```python
from build123d import *

# Parameters (mm, degrees)
SKETCH1_R           = 133.35
BOSS_EXTRUDE1_DEPTH = 19.05
SKETCH2_R           = 3.6703
SKETCH2_R_2         = 2.5781
SKETCH2_R_3         = 1.7859375
CUT_EXTRUDE1_DEPTH  = 20.05
BOSS_EXTRUDE2_DEPTH = 19.05
FILLET1_R           = 25.4
SKETCH4_R           = 3.175
CUT_EXTRUDE2_DEPTH  = 20.05
SKETCH5_R           = 7.9375
CUT_EXTRUDE3_DEPTH  = 15.875
CUT_EXTRUDE4_DEPTH  = 20.05
CUT_EXTRUDE5_DEPTH  = 12.7
FILLET2_R           = 3.175
CUT_EXTRUDE6_DEPTH  = 3.175


with BuildPart() as part:
    # Sketch1 → Boss-Extrude1 (new body)
    with BuildSketch(Plane(origin=(0, 0, 0), x_dir=(1, 0, 0), z_dir=(0, 1, 0))):
        Circle(SKETCH1_R)
    extrude(amount=BOSS_EXTRUDE1_DEPTH)

    # Sketch2 → Cut-Extrude1 (cut, through all)
    with BuildSketch(Plane(origin=(0, 19.05, 0), x_dir=(1, 0, 0), z_dir=(0, 1, 0))):
        with Locations((-120.2563, 0)):
            Circle(SKETCH2_R)
        with Locations((-111.10233558, 46.02009338)):
            Circle(SKETCH2_R_2)
        with Locations((120.2563, 0)):
            Circle(SKETCH2_R)
        with Locations((0, -120.2563)):
            Circle(SKETCH2_R)
        with Locations((0, 120.2563)):
            Circle(SKETCH2_R)
        with Locations((111.10233558, -46.02009338)):
            Circle(SKETCH2_R_2)
        with Locations((-46.02009338, -111.10233558)):
            Circle(SKETCH2_R_2)
        with Locations((46.02009338, 111.10233558)):
            Circle(SKETCH2_R_2)
        with Locations((-85.03404521, -85.03404521)):
            Circle(SKETCH2_R_3)
        with Locations((85.03404521, 85.03404521)):
            Circle(SKETCH2_R_3)
        with Locations((-85.03404521, 85.03404521)):
            Circle(SKETCH2_R_3)
        with Locations((85.03404521, -85.03404521)):
            Circle(SKETCH2_R_3)
    extrude(amount=-CUT_EXTRUDE1_DEPTH, mode=Mode.SUBTRACT)

    # Sketch3 → Boss-Extrude2 (add)
    with BuildSketch(Plane(origin=(0, 19.05, 0), x_dir=(1, 0, 0), z_dir=(0, 1, 0))):
        with BuildLine():
            Line((-106.3625, 80.431592635), (-106.3625, 188.9125))
            ThreePointArc((-106.3625, 188.9125), (-102.642756121, 197.892756121), (-93.6625, 201.6125))
            Line((-93.6625, 201.6125), (93.6625, 201.6125))
            ThreePointArc((93.6625, 201.6125), (102.642756121, 197.892756121), (106.3625, 188.9125))
            Line((106.3625, 188.9125), (106.3625, 80.431592635))
            ThreePointArc((106.3625, 80.431592635), (0, 133.35), (-106.3625, 80.431592635))
        make_face()
    extrude(amount=-BOSS_EXTRUDE2_DEPTH)

    # Fillet1
    fillet1_edges = [part.edges().sort_by_distance(p)[0] for p in [
        (106.3625, 9.525, -80.431592635),
        (-106.3625, 9.525, -80.431592635),
    ]]
    fillet(fillet1_edges, radius=FILLET1_R)

    # Sketch4 → Cut-Extrude2 (cut, through all)
    with BuildSketch(Plane(origin=(0, 19.05, 0), x_dir=(1, 0, 0), z_dir=(0, 1, 0))):
        with Locations((-93.6625, 188.9125)):
            Circle(SKETCH4_R)
        with Locations((93.6625, 188.9125)):
            Circle(SKETCH4_R)
        with Locations((93.5355, -1.5875)):
            Circle(SKETCH4_R)
        with Locations((-93.5355, -1.5875)):
            Circle(SKETCH4_R)
        with BuildLine():
            Line((-38.1, 165.1), (-38.1, 195.2625))
            ThreePointArc((-38.1, 195.2625), (-39.959871939, 199.752628061), (-44.45, 201.6125))
            Line((-44.45, 201.6125), (-6.35, 201.6125))
            ThreePointArc((-6.35, 201.6125), (-10.840128061, 199.752628061), (-12.7, 195.2625))
            Line((-12.7, 195.2625), (-12.7, 165.1))
            ThreePointArc((-12.7, 165.1), (-13.164967985, 163.977467985), (-14.2875, 163.5125))
            Line((-14.2875, 163.5125), (-36.5125, 163.5125))
            ThreePointArc((-36.5125, 163.5125), (-37.635032015, 163.977467985), (-38.1, 165.1))
        make_face()
    extrude(amount=-CUT_EXTRUDE2_DEPTH, mode=Mode.SUBTRACT)

    # Sketch5 → Cut-Extrude3 (cut)
    with BuildSketch(Plane.XZ):
        with Locations((-93.5355, 1.5875)):
            Circle(SKETCH5_R)
        with Locations((-93.6625, -188.9125)):
            Circle(SKETCH5_R)
        with Locations((93.6625, -188.9125)):
            Circle(SKETCH5_R)
        with Locations((93.5355, 1.5875)):
            Circle(SKETCH5_R)
    extrude(amount=-CUT_EXTRUDE3_DEPTH, mode=Mode.SUBTRACT)

    # Sketch6 → Cut-Extrude4 (cut, through all)
    with BuildSketch(Plane.XZ):
        with BuildLine():
            ThreePointArc((-97.25707655, -29.387430322), (0, -101.6), (97.25707655, -29.387430322))
            ThreePointArc((97.25707655, -29.387430322), (96.312482934, -19.750032603), (88.849078878, -13.580000851))
            ThreePointArc((88.849078878, -13.580000851), (77.662785938, 1.318105668), (88.337075578, 16.587233615))
            ThreePointArc((88.337075578, 16.587233615), (95.586803849, 23.006979086), (96.203812617, 32.67088058))
            ThreePointArc((96.203812617, 32.67088058), (0, 101.6), (-96.203812617, 32.67088058))
            ThreePointArc((-96.203812617, 32.67088058), (-95.586803849, 23.006979086), (-88.337075578, 16.587233615))
            ThreePointArc((-88.337075578, 16.587233615), (-77.662785938, 1.318105668), (-88.849078878, -13.580000851))
            ThreePointArc((-88.849078878, -13.580000851), (-96.312482934, -19.750032603), (-97.25707655, -29.387430322))
        make_face()
    extrude(amount=-CUT_EXTRUDE4_DEPTH, mode=Mode.SUBTRACT)

    # Sketch7 → Cut-Extrude5 (cut)
    with BuildSketch(Plane(origin=(0, 19.05, 0), x_dir=(1, 0, 0), z_dir=(0, 1, 0))):
        with BuildLine():
            Line((106.3625, 131.527748149), (9.586053414, 152.098216886))
            add(Edge.make_bspline(
                [(9.586053414, 152.098216886), (-20.233717631, 158.436604889), (-75.860757578, 134.149121206), (-106.3625, 105.832753729)],
                knots=[0, 0, 0, 0, 1, 1, 1, 1], degree=3))
            Line((-106.3625, 105.832753729), (-110.6805, 74.377748149))
            ThreePointArc((-110.6805, 74.377748149), (-108.217560682, 77.917790395), (-105.641439401, 81.376340427))
            Line((-105.641439401, 81.376340427), (-100.142178087, 84.551340427))
            ThreePointArc((-100.142178087, 84.551340427), (-56.884848889, 98.527448456), (-23.15251969, 129.001340427))
            Line((-23.15251969, 129.001340427), (-17.653258376, 132.176340427))
            ThreePointArc((-17.653258376, 132.176340427), (54.760261489, 121.58756623), (110.6805, 74.377748149))
            Line((110.6805, 74.377748149), (106.3625, 131.527748149))
        make_face()
    extrude(amount=-CUT_EXTRUDE5_DEPTH, mode=Mode.SUBTRACT)

    # Fillet2
    fillet2_edges = [part.edges().sort_by_distance(p)[0] for p in [
        (-106.3625, 12.7, -105.832753729),
        (106.3625, 12.7, -131.527748149),
    ]]
    fillet(fillet2_edges, radius=FILLET2_R)

    # Sketch8 → Cut-Extrude6 (cut)
    with BuildSketch(Plane(origin=(0, 19.05, 0), x_dir=(1, 0, 0), z_dir=(0, 1, 0))):
        with BuildLine():
            Line((27.78125, 115.8875), (-11.90625, 115.8875))
            ThreePointArc((-11.90625, 115.8875), (-13.590048023, 115.190048023), (-14.2875, 113.50625))
            Line((-14.2875, 113.50625), (-14.2875, 84.1375))
            Line((-14.2875, 84.1375), (30.1625, 84.1375))
            Line((30.1625, 84.1375), (30.1625, 113.50625))
            ThreePointArc((30.1625, 113.50625), (29.465048023, 115.190048023), (27.78125, 115.8875))
        make_face()
    extrude(amount=-CUT_EXTRUDE6_DEPTH, mode=Mode.SUBTRACT)


solid = part.part
```
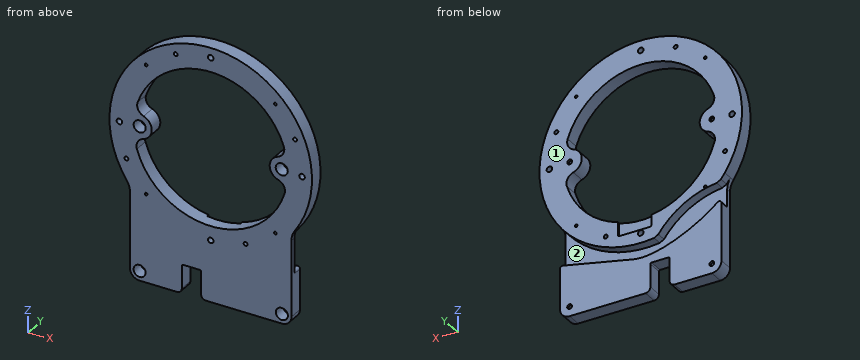
Here's how the part is built. I have some questions about the finished solid (model axes, mm). Face numbers are marked on the shaded views. Round coordinates to 2 decimals unless told otherwise and drop trailing zeros. Loops run counter-clockwise (first coordinate to the right, second up) from the corner with the lowest first, then second, coordinate; pieces in that order, holes last. Notation, with made-up numbers: (-4.5, 89.5) -> (50.5, 89.5) arc R22 ccw to (50.5, 117.5) -> close; hole circle Ø11 at (31.25, -1.5). An arc over 180 degrees is marked (long way). Answer as CSV lines item,"result". Start each with the question number.
1. Imagine slicing it at A-A on z = -54. Write out the boundary of the cut face in (x, y).
2. Imagine slicing it at B-B on y = 9.75. State how many separate pieces and enclosed holes the cut face has, plus the area to 3 significant figures.
3. I'm going to push flat-ended pins straight in: P1, Ø5.5, axis at y = 13.5, z = -179.5, coming from the -X side; P2, Ø1.6, axis at y = 17, z = -109, coming from the +X side; P3, Ø8, axis at x = -93, z = 4, coming from the -Y side (3 decimals); P4, Ø12, axis at x = 84, z = -33.5, coming from the +Y side. Where does each tip first touch, or does it pass through?
4. If we mould it in two halves opening along X, with no side actions, what happens to the marked faces 1 and 2? For each: pulls with the +X half, pulls with the -X half, needs draft (parallel to the pull), parting line crosses it, or undercut.
5. I need wall thicknesses on probe 1 along X at (y, z) = (14.25, -170.5); probe 2 along Z at (x, y) = (8.5, 17.75); probe 3 along Z at (x, y) = (69.5, 8.5). Which ranges of each line are inside material? Lowest first, please. Write a range as from..to.
Solution:
1,outline,"(-121.93, 0) -> (-86.06, 0) -> (-86.06, 19.05) -> (-121.93, 19.05) -> close; (86.06, 0) -> (121.93, 0) -> (121.93, 19.05) -> (86.06, 19.05) -> close"
2,separate pieces,"2"
2,enclosed holes,"17"
2,area,"34,700 mm²"
3,P1,"x = -106.36"
3,P2,"x = 77.94"
3,P3,"y = 15.875"
3,P4,"through"
4,face 1,"needs draft"
4,face 2,"undercut"
5,probe 1,"-106.36..-38.1, -12.7..106.36"
5,probe 2,"-201.61..-152.31, -133.08..-115.89, 101.24..133.08"
5,probe 3,"-201.61..-139.36, -113.81..-74.11, 74.11..113.81"
